Verification items for the finished model (mm, model axes). Face numbers are marked on the shaded views. A direction names the side the tool comes from. Round coordinates to 2 decimals unless told otherwise and drop trailing zeros. Order: outer loops, then holes, each group sorted by start corner. A loop starts at its lowest first (then second) coordinate and runs counter-clockwise, first axis right, second up. Notation, with made-up numbers: M 87,9.5 L 102,9.5 A13 cw 102,14.5 Z; hole C 16.25,3 d3. An arc over 180 degrees is marked long. Use one line per item in the form item = value. Start each with the question number.
Item 1: Tool access check on the marked faces 1 and 2. Record the directions out of +Z, -Z, +X, -X, +Y, -Y that give a thin tool (end or side, any length) a straight path to the whole face; none if there is none.
Item 2: Release check for a two-part mould opening along Z. For the marked faces 3, 4 and 5 record: +Z half, -Z half, draft (parallel to the pull), parting line (faces both ways), or undercut.
Item 3: Cross-section at C-C on x = -6.5. Enter the section's corners in (y, z) (3 decimals), then the cut area to 3 significant figures.
Item 4: Go/stop test with flat-tipped pins: pin 1 Ø8 at (x, z) = (-14.5, -21.5) entering from -Y; pin 2 Ø8 at (x, z) = (-11, -5) entering from +Y; pin 3 Ø1 at (x, z) = (-12, -4) entering from +Y. Record where each tip stops, or that it passes through.
Item 5: Cross-section at B-B on y = 184. Enter the section's corners in (x, z) (3 decimals), then the cut area to 3 significant figures.
Item 6: Cross-section at A-A on z = -5.75. Enter the section's corners in (x, y) (3 decimals), then the cut area to 3 significant figures.
Item 7: Thickness scan on probe 1 along Y at (x, z) = (-25.4, -1.5); probe 2 along Z at (x, y) = (-6, 80.5) (3 decimals); probe 3 along X at (y, z) = (149, -15.25) (3 decimals). Record the ranges inside material, lowest first. Write a range as [from, to].
Item 8: Cross-section at D-D on y = 32. Enter the section's corners in (x, z) (3 decimals).
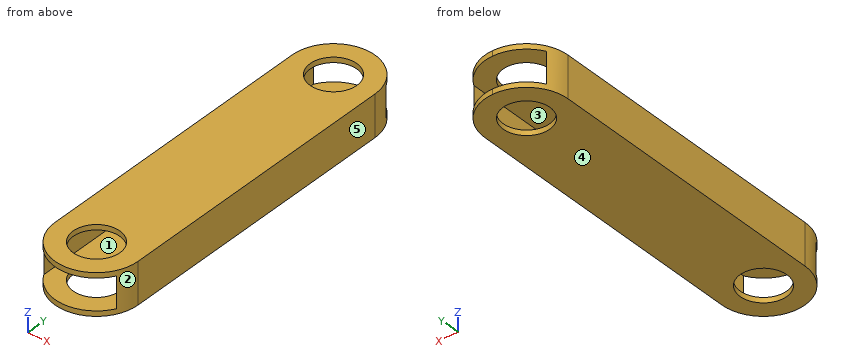
Autodesk Inventor part; units mm, degrees
ref_plane "YZ Plane" through (0, 0, 0) normal (1, 0, 0) x (0, 1, 0)
ref_plane "XZ Plane" through (0, 0, 0) normal (0, 1, 0) x (-1, 0, 0)
ref_plane "XY Plane" through (0, 0, 0) normal (0, 0, 1) x (1, 0, 0)
sketch "Sketch1" plane through (0, 0, 0) normal (0, 1, 0) x (-1, 0, 0)
  line L0 (0, 0) -> (50.8, 0)
  line L1 (50.8, 0) -> (50.8, -25.4)
  line L2 (50.8, -25.4) -> (0, -25.4)
  line L3 (0, -25.4) -> (0, 0)
  line L4 (47.625, -22.225) -> (47.625, -3.175)
  line L5 (47.625, -3.175) -> (3.175, -3.175)
  line L6 (3.175, -3.175) -> (3.175, -22.225)
  line L7 (3.175, -22.225) -> (47.625, -22.225)
  dimension "d0" = 50.8
  dimension "d1" = 25.4
  dimension "d2" = 3.175
extrude "Extrusion1" add sketch "Sketch1" along normal blind 228.6
sketch "Sketch2" plane through (0, 0, -25.4) normal (0, 0, -1) x (-1, 0, 0)
  line L0 (50.8, 0) -> (0, 0)
  line L1 (50.8, 0) -> (50.8, 228.6)
  line L2 (0, 228.6) -> (50.8, 228.6)
  line L3 (0, 0) -> (0, 228.6)
  circle A0 centre (25.4, 203.2) radius 14.2875
  circle A1 centre (25.4, 25.4) radius 14.2875
  dimension "d5" = 25.4
  dimension "d6" = 25.4
  dimension "d7" = 28.575
  dimension "d8" = 25.4
  dimension "d9" = 25.4
  dimension "d10" = 28.575
extrude "Extrusion2" cut sketch "Sketch2" against normal through all contours A0 | A1
fillet "Fillet1" radius 25.4 4 edges at (-50.8, 228.6, -12.7) (0, 228.6, -12.7) (-50.8, 0, -12.7) (0, 0, -12.7)
properties part number "WristBarr.ver1-1111-2020"
Output values:
q1.face_1 = +Y, -Y
q1.face_2 = +Z, -Z, -Y
q2.face_3 = undercut
q2.face_4 = -Z half
q2.face_5 = draft
q3.outline = M 8.431,-25.4 L 220.169,-25.4 L 220.169,-22.225 L 8.431,-22.225 Z; M 8.431,-3.175 L 220.169,-3.175 L 220.169,0 L 8.431,0 Z
q3.area = 1,340 mm2
q4.pin_1 = 0.97
q4.pin_2 = 226.17
q4.pin_3 = through
q5.outline = M -50.8,-25.4 L 0,-25.4 L 0,0 L -50.8,0 Z; hole M -47.625,-22.225 L -3.175,-22.225 L -3.175,-3.175 L -47.625,-3.175 Z
q5.area = 444 mm2
q6.outline = M -50.8,25.4 A25.4 ccw -47.625,13.103 L -47.625,215.497 A25.4 ccw -50.8,203.2 Z; M -3.175,13.103 A25.4 ccw 0,25.4 L 0,203.2 A25.4 ccw -3.175,215.497 Z
q6.area = 1,230 mm2
q7.probe_1 = [0, 11.11], [39.69, 188.91], [217.49, 228.6]
q7.probe_2 = [-25.4, -22.225], [-3.175, 0]
q7.probe_3 = [-50.8, -47.625], [-3.175, 0]
q8.outline = M -50.8,-25.4 L -38.072,-25.4 L -38.072,-22.225 L -47.625,-22.225 L -47.625,-3.175 L -38.072,-3.175 L -38.072,0 L -50.8,0 Z; M -12.728,-25.4 L 0,-25.4 L 0,0 L -12.728,0 L -12.728,-3.175 L -3.175,-3.175 L -3.175,-22.225 L -12.728,-22.225 Z
